```python
from build123d import *

# Parameters (mm, degrees)
BOSS_EXTRUDE1_DEPTH = 12.7
BOSS_EXTRUDE2_DEPTH = 19.05
SKETCH6_W           = 12.7
SKETCH6_H           = 12.7
BOSS_EXTRUDE3_DEPTH = 25.4
SKETCH6_3_W         = 12.7
SKETCH6_3_H         = 38.1
BOSS_EXTRUDE4_DEPTH = 6.35
FILLET1_R           = 6.35


with BuildPart() as part:
    # Sketch1 → Boss-Extrude1 (new body)
    with BuildSketch(Plane(origin=(0, 0, 0), x_dir=(1, 0, 0), z_dir=(0, 1, 0))):
        with BuildLine():
            Line((82.55, 63.5), (50.8, 63.5))
            Line((50.8, 63.5), (50.8, 31.749999876))
            ThreePointArc((50.8, 31.749999876), (60.099359653, 54.200640259), (82.55, 63.5))
        make_face()
        with BuildLine():
            ThreePointArc((82.55, 0), (60.099359741, 9.299359653), (50.8, 31.749999876))
            Line((50.8, 31.749999876), (50.8, 0))
            Line((50.8, 0), (82.55, 0))
        make_face()
        with BuildLine():
            ThreePointArc((82.55, 63.5), (60.099359653, 54.200640259), (50.8, 31.749999876))
            ThreePointArc((50.8, 31.749999876), (60.099359741, 9.299359653), (82.55, 0))
            Line((82.55, 0), (82.55, 22.225))
            ThreePointArc((82.55, 22.225), (73.025, 31.75), (82.55, 41.275))
            Line((82.55, 41.275), (82.55, 63.5))
        make_face()
        with BuildLine():
            ThreePointArc((114.3, 31.75), (105.000640303, 54.200640303), (82.55, 63.5))
            Line((82.55, 63.5), (82.55, 41.275))
            ThreePointArc((82.55, 41.275), (89.285192091, 38.485192091), (92.075, 31.75))
            ThreePointArc((92.075, 31.75), (89.285192091, 25.014807909), (82.55, 22.225))
            Line((82.55, 22.225), (82.55, 0))
            ThreePointArc((82.55, 0), (105.000640303, 9.299359697), (114.3, 31.75))
        make_face()
    extrude(amount=BOSS_EXTRUDE1_DEPTH)

    # Sketch1_4 → Boss-Extrude2 (add)
    with BuildSketch(Plane(origin=(0, 0, 0), x_dir=(1, 0, 0), z_dir=(0, 1, 0))):
        Polygon((50.8, 31.749999876), (50.8, 63.5), (0, 63.5), (0, 0), (50.8, 0), align=None)
    extrude(amount=BOSS_EXTRUDE2_DEPTH)

    # Sketch6 → Boss-Extrude3 (add)
    with BuildSketch(Plane(origin=(0, 19.05, 0), x_dir=(1, 0, 0), z_dir=(0, 1, 0))):
        with Locations((6.35, 57.15)):
            Rectangle(SKETCH6_W, SKETCH6_H)
        with Locations((6.35, 6.35)):
            Rectangle(SKETCH6_W, SKETCH6_H)
        with Locations((44.45, 57.15)):
            Rectangle(SKETCH6_W, SKETCH6_H)
        with Locations((44.45, 6.35)):
            Rectangle(SKETCH6_W, SKETCH6_H)
    extrude(amount=BOSS_EXTRUDE3_DEPTH)

    # Sketch6_3 → Boss-Extrude4 (add)
    with BuildSketch(Plane(origin=(0, 19.05, 0), x_dir=(1, 0, 0), z_dir=(0, 1, 0))):
        with Locations((6.35, 31.75)):
            Rectangle(SKETCH6_3_W, SKETCH6_3_H)
        with Locations((44.45, 31.75)):
            Rectangle(SKETCH6_3_W, SKETCH6_3_H)
    extrude(amount=BOSS_EXTRUDE4_DEPTH)

    # Fillet1
    fillet1_edges = [part.edges().sort_by_distance(p)[0] for p in [
        (50.8, 12.7, -31.75),
    ]]
    fillet(fillet1_edges, radius=FILLET1_R)


solid = part.part
```
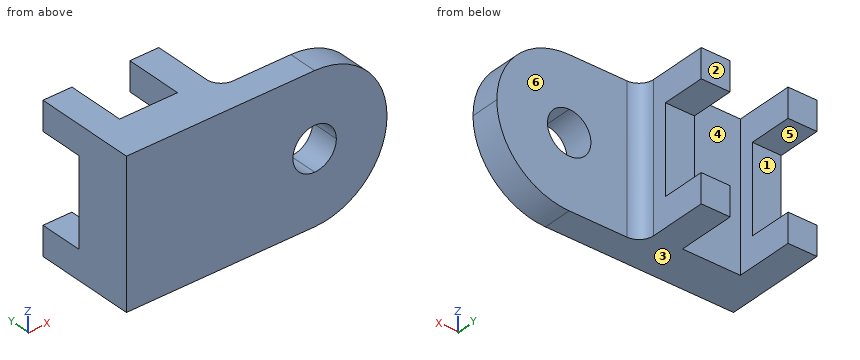
The model under review builds one solid part; all positions refer to its coordinate system, in mm. Face numbers are marked on the shaded views. A direction names the side the tool comes from. Round coordinates to 2 decimals unless told otherwise and drop trailing zeros. Loops run counter-clockwise (first coordinate to the right, second up) from the corner with the lowest first, then second, coordinate; pieces in that order, holes last. Notation, with made-up numbers: M 1.25,-7.75 L 47.25,-7.75 A26 ccw 47.25,21.25 Z; hole C 66,-19 d8. An arc over 180 degrees is marked long. Put each result on its own line as item: value.
Q1. Machinability: for the marked faces 4, 5 and 6, which of the approach directions +Z, -Z, +X, -X, +Y, -Y give a long, thin tool a straight path to every point of the face, cutting with its end or side? Answer none if there is none.
Result set:
face 4: +Z, -Z, +Y
face 5: +X, -X, +Y
face 6: +Z, -Z, +X, +Y
Q2. Consider section A-A, the plane y = 11. Give the boundary of the cut face in (x, z) (3 decimals), then the cut area to 3 significant figures.
Result set:
outline: M 0,-63.5 L 82.55,-63.5 A31.75 ccw 82.55,0 L 0,0 Z; hole C 82.55,-31.75 d19.05
area: 6,540 mm²
Q3. Mouldability with a two-part tool opening along Z and no side actions: class the marked faces 1, 2 and 3 as released by +Z, released by -Z, zero draft, split by the parting line, or undercut.
Result set:
face 1: undercut
face 2: zero draft
face 3: released by -Z
Q4. To check wall thickness, follow L1, parallel to X at y = 36.5, z = -9; L2, parallel to Z at x = 47, y = 28.5; L3, parallel to Y at x = 62.5, z = -29.5. State the ranges of each line that lie inside material, in increasing order.
Result set:
L1: x = 0 to 12.7, 38.1 to 50.8
L2: z = -63.5 to -50.8, -12.7 to 0
L3: y = 0 to 12.7
Q5. Consider section D-D, the plane z = -45.5. Give the boundary of the cut face in (x, y), then the cut area to 3 significant figures.
Result set:
outline: M 0,0 L 111.17,0 L 111.17,12.7 L 57.15,12.7 A6.35 cw 50.8,19.05 L 50.8,25.4 L 38.1,25.4 L 38.1,19.05 L 12.7,19.05 L 12.7,25.4 L 0,25.4 Z
area: 1,900 mm²
Q6. For pin 1 (3 mm diameter, centred on x = 20, z = -27, fed in from -Y); pin 2 (14 mm diameter, centred on x = 44.5, z = -24.5, fed in from +Y); pin 3 (8 mm diameter, centred on y = 26.5, z = -9, fed in from +X); pin 4 (10 mm diameter, centred on x = 77, z = -38, fed in from +Y), all flat-tipped, find the tip position at first contact; note any pin that passes through.
Result set:
pin 1: stops at y = 0
pin 2: stops at y = 25.4
pin 3: stops at x = 50.8
pin 4: stops at y = 12.7
Q7. Consider section C-C, the plane x = 43.5. Give the boundary of the cut face in (y, z), then the cut area to 3 significant figures.
Result set:
outline: M 0,-63.5 L 44.45,-63.5 L 44.45,-50.8 L 25.4,-50.8 L 25.4,-12.7 L 44.45,-12.7 L 44.45,0 L 0,0 Z
area: 2,100 mm²
Q8. Consider section B-B, the plane y = 35. Give the boundary of the cut face in (x, z).
Result set:
outline: M 0,-63.5 L 12.7,-63.5 L 12.7,-50.8 L 0,-50.8 Z; M 0,-12.7 L 12.7,-12.7 L 12.7,0 L 0,0 Z; M 38.1,-63.5 L 50.8,-63.5 L 50.8,-50.8 L 38.1,-50.8 Z; M 38.1,-12.7 L 50.8,-12.7 L 50.8,0 L 38.1,0 Z
